Could you check a few things on this model? Use its own coordinates, in mm. A direction names the side the tool comes from. Coordinates: 2 decimals unless noted, no trailing zeros. Write each loop counter-clockwise with the first axis right and the second up, starting at its lowest first coordinate (ties: lowest second). Pieces come first, ordered by that corner, then holes. Notation, with made-up numbers: (69, 86.5) - (116, 86.5) arc R19 ccw to (116, 112.5) - close; hole circle Ø6 at (23.25, 29). An arc over 180 degrees is marked (long way). Answer as a JSON object with one key per item and string values. Group by question number.
1) If we section it at A-A (z = -10.25): Write out the boundary of the cut face in (x, y).
2) On a 3-axis mill with a long thin cutter (end or side, diameter ignored), from which of +Z, -Z, +X, -X, +Y, -Y can I reach the whole of each face in a straight line? I mean faces 1 (the flat face through (0, -11, 12)), 2 (the flat face through (0, 15, 5)), 3 (the flat face through (-21, 29, -6)), 4 (the cylindrical face through (10.24, 2.39, 12.01)), 5 (the flat face through (0, 0, 11)). Say none if no direction works.
3) If we section it at C-C (x = -9): Write out the boundary of the cut face in (y, z), plus the area to 3 significant figures.
4) If we section it at B-B (y = 2): Write out the boundary of the cut face in (x, z), plus the area to 3 significant figures.
5) If we section it at D-D (y = 9.5): Write out the boundary of the cut face in (x, z), plus the area to 3 significant figures.
6) Will these pins go through, and if not, where does the flat tip stop? pin 1 Ø10 at (x, y) = (14.5, 6) entering from -Z; pin 2 Ø6 at (y, z) = (6, 5.5) entering from -X; pin 3 Ø1.5 at (x, y) = (-18, 25.5) entering from -Z; pin 4 Ø7.5 at (x, z) = (-2, -5.5) entering from +Y.
7) We'd pull the mould along Y, two halves only. Please class faces 6 (the cylindrical face through (10.2, -9.5, 12)), 7 (the cylindrical face through (-7.8, -9.5, 12)), 8 (the flat face through (-11, 7.1, 11.3)), 9 (the flat face through (0, -28, -9)): released by +Y, released by -Y, zero draft, split by the parting line, or undercut.
8) Please list where these lines run through material, in increasing order: line 1 along Y through (x, z) = (-23.5, -0.95); line 2 along Z through (x, y) = (8.5, -7); line 3 along Z through (x, y) = (1, -1.5).
```python
from build123d import *

# Parameters (mm, degrees)
SKETCH_1_W          = 50
SKETCH_1_H          = 70
EXTRUDE_1_DEPTH     = 1.5
SKETCH_2_R          = 1
CUT_EXTRUDE_1_DEPTH = 1.5
SKETCH_3_W          = 50
SKETCH_3_H          = 18
EXTRUDE_2_DEPTH     = 15
EXTRUDE_3_DEPTH     = 15
SKETCH_5_W          = 7
SKETCH_5_H          = 10
EXTRUDE_4_DEPTH     = 10
EXTRUDE_5_DEPTH     = 13
SKETCH_7_W          = 22
SKETCH_7_H          = 11
CUT_EXTRUDE_2_DEPTH = 23
CUT_EXTRUDE_3_DEPTH = 2
SKETCH_9_W          = 10
SKETCH_9_H          = 10
CUT_EXTRUDE_4_DEPTH = 0.5
SKETCH_10_W         = 10
SKETCH_10_H         = 10
CUT_EXTRUDE_5_DEPTH = 0.5
CUT_EXTRUDE_6_REACH = 54.156
SKETCH_11_R         = 1.3
SKETCH_12_W         = 5
SKETCH_12_H         = 4.5
CUT_EXTRUDE_8_DEPTH = 0.1


with BuildPart() as part:
    # 草图1 → 凸台-拉伸1 (new body)
    with BuildSketch(Plane.XY):
        Rectangle(SKETCH_1_W, SKETCH_1_H)
    extrude(amount=-EXTRUDE_1_DEPTH)

    # 草图2 → 切除-拉伸1 (cut)
    with BuildSketch(Plane.XY):
        with Locations((-23.5, 33.5)):
            Circle(SKETCH_2_R)
        with Locations(Location((23.5, 33.5, 0), (0, 0, 180))):
            Circle(SKETCH_2_R)
        with Locations((23.5, -33.5)):
            Circle(SKETCH_2_R)
        with Locations(Location((-23.5, -33.5, 0), (0, 0, 180))):
            Circle(SKETCH_2_R)
    extrude(amount=-CUT_EXTRUDE_1_DEPTH, mode=Mode.SUBTRACT)

    # 草图3 → 凸台-拉伸2 (add)
    with BuildSketch(Plane(origin=(0, 0, -1.5), x_dir=(-1, 0, 0), z_dir=(0, 0, -1))):
        with Locations((0, -19)):
            Rectangle(SKETCH_3_W, SKETCH_3_H)
    extrude(amount=EXTRUDE_2_DEPTH)

    # 草图4 → 凸台-拉伸3 (add)
    with BuildSketch(Plane(origin=(0, 0, -1.5), x_dir=(-1, 0, 0), z_dir=(0, 0, -1))):
        Polygon((-8, -2), (0, -2), (8, -2), (8, 12), (-8, 12), align=None)
    extrude(amount=EXTRUDE_3_DEPTH)

    # 草图5 → 凸台-拉伸4 (add)
    with BuildSketch(Plane(origin=(0, 0, -1.5), x_dir=(-1, 0, 0), z_dir=(0, 0, -1))):
        with Locations((-21.5, 24)):
            Rectangle(SKETCH_5_W, SKETCH_5_H)
        with Locations((21.5, 24)):
            Rectangle(SKETCH_5_W, SKETCH_5_H)
    extrude(amount=EXTRUDE_4_DEPTH)

    # 草图6 → 凸台-拉伸5 (add)
    with BuildSketch(Plane.XY):
        Polygon((0, 17), (11, 17), (11, -11), (-11, -11), (-11, 17), align=None)
    extrude(amount=EXTRUDE_5_DEPTH)

    # 草图7 → 切除-拉伸2 (cut)
    with BuildSketch(Plane(origin=(0, -11, 0), x_dir=(-1, 0, 0), z_dir=(0, -1, 0))):
        with Locations((0, -5.5)):
            Rectangle(SKETCH_7_W, SKETCH_7_H)
    extrude(amount=-CUT_EXTRUDE_2_DEPTH, mode=Mode.SUBTRACT)

    # 草图8 → 切除-拉伸3 (cut)
    with BuildSketch(Plane(origin=(0, 17, 0), x_dir=(1, 0, 0), z_dir=(0, 1, 0))):
        Polygon((0, 0), (11, 0), (11, -11), (-11, -11), (-11, 0), align=None)
    extrude(amount=-CUT_EXTRUDE_3_DEPTH, mode=Mode.SUBTRACT)

    # 草图9 → 切除-拉伸4 (cut)
    with BuildSketch(Plane.ZY.offset(25)):
        with Locations((-6.5, 24)):
            Rectangle(SKETCH_9_W, SKETCH_9_H)
    extrude(amount=-CUT_EXTRUDE_4_DEPTH, mode=Mode.SUBTRACT)

    # 草图10 → 切除-拉伸5 (cut)
    with BuildSketch(Plane(origin=(25, 0, 0), x_dir=(0, 0, -1), z_dir=(1, 0, 0))):
        with Locations((6.5, 24)):
            Rectangle(SKETCH_10_W, SKETCH_10_H)
    extrude(amount=-CUT_EXTRUDE_5_DEPTH, mode=Mode.SUBTRACT)

    # 草图11 → 切除-拉伸6 (cut, up to next)
    with BuildSketch(Plane.XY.offset(13), mode=Mode.PRIVATE) as cut_extrude_6_sk1:
        with Locations((-9, 2)):
            Circle(SKETCH_11_R)
    cut_extrude_6_tool1 = extrude(cut_extrude_6_sk1.sketch, amount=-CUT_EXTRUDE_6_REACH, mode=Mode.PRIVATE) & part.part
    # 草图11 → 切除-拉伸6 (cut, up to next)
    with BuildSketch(Plane.XY.offset(13), mode=Mode.PRIVATE) as cut_extrude_6_sk2:
        with Locations((-9, -9)):
            Circle(SKETCH_11_R)
    cut_extrude_6_tool2 = extrude(cut_extrude_6_sk2.sketch, amount=-CUT_EXTRUDE_6_REACH, mode=Mode.PRIVATE) & part.part
    # 草图11 → 切除-拉伸6 (cut, up to next)
    with BuildSketch(Plane.XY.offset(13), mode=Mode.PRIVATE) as cut_extrude_6_sk3:
        with Locations((9, 2)):
            Circle(SKETCH_11_R)
    cut_extrude_6_tool3 = extrude(cut_extrude_6_sk3.sketch, amount=-CUT_EXTRUDE_6_REACH, mode=Mode.PRIVATE) & part.part
    # 草图11 → 切除-拉伸6 (cut, up to next)
    with BuildSketch(Plane.XY.offset(13), mode=Mode.PRIVATE) as cut_extrude_6_sk4:
        with Locations((9, -9)):
            Circle(SKETCH_11_R)
    cut_extrude_6_tool4 = extrude(cut_extrude_6_sk4.sketch, amount=-CUT_EXTRUDE_6_REACH, mode=Mode.PRIVATE) & part.part
    add(cut_extrude_6_tool1.solids().sort_by_distance((-9, 2, 13))[0], mode=Mode.SUBTRACT)
    add(cut_extrude_6_tool2.solids().sort_by_distance((-9, -9, 13))[0], mode=Mode.SUBTRACT)
    add(cut_extrude_6_tool3.solids().sort_by_distance((9, 2, 13))[0], mode=Mode.SUBTRACT)
    add(cut_extrude_6_tool4.solids().sort_by_distance((9, -9, 13))[0], mode=Mode.SUBTRACT)

    # 草图12 → 切除-拉伸8 (cut)
    with BuildSketch(Plane.XY.offset(13)):
        with Locations((0, -3.5)):
            Rectangle(SKETCH_12_W, SKETCH_12_H)
    extrude(amount=-CUT_EXTRUDE_8_DEPTH, mode=Mode.SUBTRACT)


solid = part.part
```
Here are the results:
{
 "1": {"outline": "(-25, -28) - (25, -28) - (25, -10) - (-25, -10) - close; (-24.5, 19) - (-18, 19) - (-18, 29) - (-24.5, 29) - close; (-8, -2) - (8, -2) - (8, 12) - (-8, 12) - close; (18, 19) - (24.5, 19) - (24.5, 29) - (18, 29) - close"},
 "2": {"face 1": "+Z, +X, -X, -Y", "face 2": "+X, -X, +Y", "face 3": "-Z, +X, -X, +Y", "face 4": "+Z", "face 5": "+X, -X, -Y"},
 "3": {"outline": "(-35, -1.5) - (-28, -1.5) - (-28, -16.5) - (-10, -16.5) - (-10, -1.5) - (35, -1.5) - (35, 0) - (15, 0) - (15, 11) - (17, 11) - (17, 13) - (3.3, 13) - (3.3, 11) - (12, 11) - (12, 0) - (-35, 0) - close; (-11, 11) - (-10.3, 11) - (-10.3, 13) - (-11, 13) - close; (-7.7, 11) - (0.7, 11) - (0.7, 13) - (-7.7, 13) - close", "area": "454 mm²"},
 "4": {"outline": "(-25, -1.5) - (-8, -1.5) - (-8, -16.5) - (8, -16.5) - (8, -1.5) - (25, -1.5) - (25, 0) - (-25, 0) - close; (-11, 11) - (-10.3, 11) - (-10.3, 13) - (-11, 13) - close; (-7.7, 11) - (7.7, 11) - (7.7, 13) - (-7.7, 13) - close; (10.3, 11) - (11, 11) - (11, 13) - (10.3, 13) - close", "area": "349 mm²"},
 "5": {"outline": "(-25, -1.5) - (-8, -1.5) - (-8, -16.5) - (8, -16.5) - (8, -1.5) - (25, -1.5) - (25, 0) - (-25, 0) - close; (-11, 11) - (11, 11) - (11, 13) - (-11, 13) - close", "area": "359 mm²"},
 "6": {"pin 1": "stops at z = -1.5", "pin 2": "passes through", "pin 3": "stops at z = -11.5", "pin 4": "stops at y = 12"},
 "7": {"face 6": "undercut", "face 7": "undercut", "face 8": "zero draft", "face 9": "released by -Y"},
 "8": {"line 1": "y = -35 to -34.5, -32.5 to 32.5, 34.5 to 35", "line 2": "z = -1.5 to 0, 11 to 13", "line 3": "z = -16.5 to 0, 11 to 12.9"}
}
